Can you work these out from the drawing? Everything is in mm from the part's minimum corner. Round coordinates to 2 decimals unless told otherwise and drop trailing zeros. Order: outer loops, then holes, each group sorted by start corner. A loop starts at its lowest first (then second) coordinate and runs counter-clockwise, first axis right, second up. Notation, with made-up numbers: M 14,23.25 L 29,23.25 A28 cw 29,51.25 Z; hole C -37.75,-38 d3. An arc over 180 degrees is marked long. Answer as CSV lines item,"result". Start each with the question number.
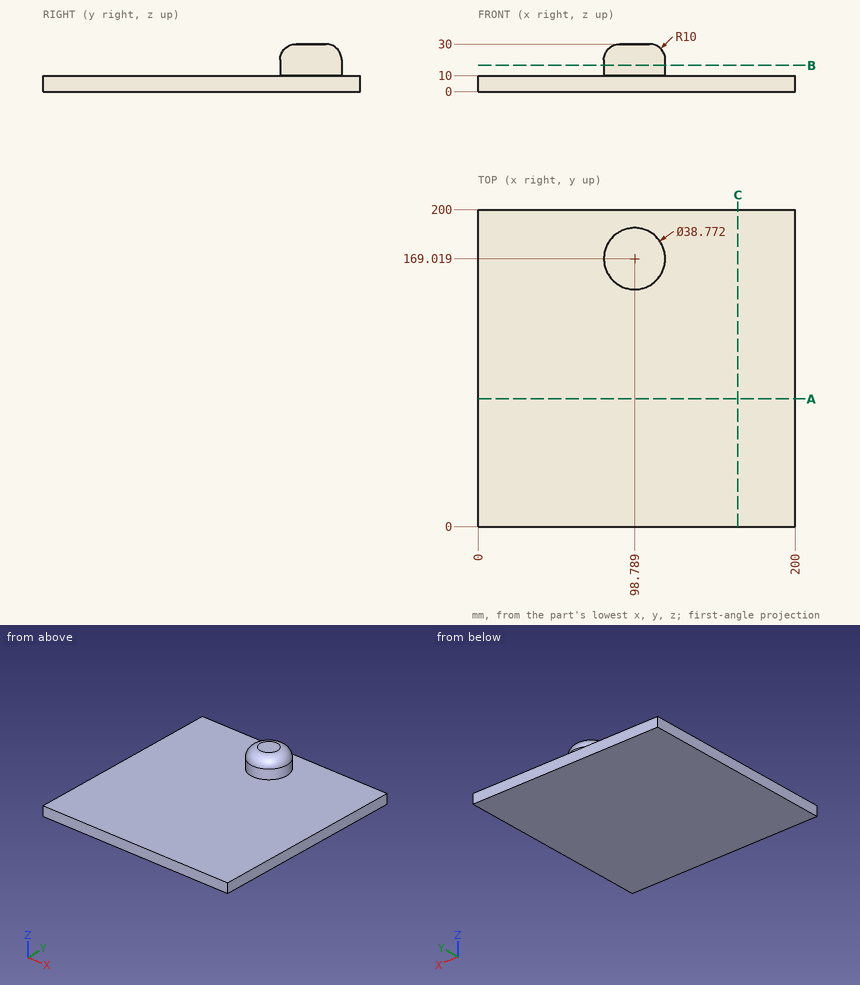
(1) I want a section at B-B on z = 16.5. Write out the boundary of the cut face in (x, y) (1 decimal).
(2) If I drill on line 1 along Z through (x, y) = (160, 30.5); line 2 along Y through (x, z) = (89, 26.75); line 3 along X through (y, z) = (167, 23), over which ranges is the centre line in solid material (lowest first)?
(3) I'm going to push flat-ended pins straight in: P1, Ø2, axis at x = 99, z = 13.5, coming from the +Y side (1 decimal); P2, Ø3, axis at x = 70, y = 177, coming from the +Z side. Where does each tip first touch, or does it pass through?
(4) I want a section at A-A on y = 80.5. Write out the boundary of the cut face in (x, z).
From the geometry:
1,outline,"C 98.8,169 d38.8"
2,line 1,"0 to 10"
2,line 2,"155.41 to 182.63"
2,line 3,"79.97 to 117.61"
3,P1,"y = 188.4"
3,P2,"z = 10"
4,outline,"M 0,0 L 200,0 L 200,10 L 0,10 Z"
